Autodesk Inventor part; units mm, degrees
ref_plane "Work Plane1" through (0, 3, 0) normal (0, -1, 0) x (1, 0, 0)
ref_plane "YZ Plane" through (0, 0, 0) normal (1, 0, 0) x (0, 1, 0)
ref_plane "XZ Plane" through (0, 0, 0) normal (0, 1, 0) x (-1, 0, 0)
sketch "Sketch1" plane through (0, 0, 0) normal (1, 0, 0) x (0, 1, 0)
  line L0 (0, 0) -> (0, -4.7)
  line L1 (0, 0) -> (3, 0)
  arc A0 (0, -4.7) -> (3, 0) centre (-2.1737, -0.0051) ccw
  dimension "d0" = 4.7
  dimension "d1" = 3
revolve "Revolution1" add sketch "Sketch1" angle 360 about axis through (0, 0, 0) along (0, 1, 0)
sketch "Sketch2" plane through (0, 0, 0) normal (0, -1, 0) x (1, 0, 0)
  circle A0 centre (0, 0) radius 2.5
  dimension "d3" = 5
extrude "Extrusion1" add sketch "Sketch2" along normal blind 12.8
thread "Thread1"
ref_plane "Work Plane1" through (0, 3, 0) normal (0, -1, 0) x (1, 0, 0)
sketch "Sketch3" plane through (0, 3, 0) normal (0, -1, 0) x (1, 0, 0)
  line L0 (0, 0) -> (0, -1.575)
  circle A0 centre (0, 0) radius 2.5
  line L1 (-0.9093, -1.575) -> (-1.8187, 0)
  line L2 (-1.8187, 0) -> (-0.9093, 1.575)
  line L3 (-0.9093, 1.575) -> (0.9093, 1.575)
  line L4 (0.9093, 1.575) -> (1.8187, 0)
  line L5 (1.8187, 0) -> (0.9093, -1.575)
  line L6 (0.9093, -1.575) -> (-0.9093, -1.575)
  dimension "d9" = 1.575
extrude "Extrusion2" cut sketch "Sketch3" along normal blind 2 contours L1 L2 L3 L4 L5 L6
properties part number "Screw"
The listing builds one solid part. Answer for the finished solid, in the listing's coordinates (mm). A direction names the side the tool comes from. Give positions to 0.01 mm unless a question says otherwise; leave off trailing zeros.
Item 1: Find the intervals of material crossed by line 1 along Y through (x, z) = (0.5, -0.25); line 2 along Y through (x, z) = (3, 2.5); line 3 along X through (y, z) = (1.5, -2), in increasing order.
Derived:
line 1: y = -12.8 to 1
line 2: y = 0 to 1.23
line 3: x = -3.05 to 3.05
Item 2: Each of these flat-tipped pins is pushed along its axis until it touches: pin 1 Ø1.9 at (x, y) = (-0.5, 1.5) entering from -Z; pin 2 Ø4 at (y, z) = (-2.5, -3) entering from +X; pin 3 Ø1.9 at (x, y) = (-0.5, 1.5) entering from +Z. Where does it stop, or does it pass through?
Derived:
pin 1: stops at z = -4.38
pin 2: stops at x = 2.29
pin 3: stops at z = 4.38
Item 3: A tool of negligible diameter and unlimited length cuts with its end or side. For faces 5 (the flat face through (1.358, 1.89, 0.799)), 6 (the flat face through (0, -12.8, 0)), from which of +Z, -Z, +X, -X, +Y, -Y can it reach the whole face along a straight path? Write none if from no direction.
Derived:
face 5: +Y
face 6: +Z, -Z, +X, -X, -Y
Item 4: Determine the mould class of faces 1 (the cylindrical face through (-0.54, -6.31, 2.44)), 2 (the flat face through (0, 2, 1.575)), 3 (the flat face through (1.37, 1.89, -0.78)), 4 (the flat face through (2, 0, -2)) for opening direction Z: +Z half, -Z half, draft (parallel to the pull), parting line (faces both ways), or undercut.
Derived:
face 1: parting line
face 2: undercut
face 3: undercut
face 4: draft
